Build history of the part. All positions in model axes, mm. Round coordinates to 2 decimals unless told otherwise and drop trailing zeros. Write each loop counter-clockwise with the first axis right and the second up, starting at its lowest first coordinate (ties: lowest second). Pieces come first, ordered by that corner, then holes. Notation, with made-up numbers: (3, 52.5) -> (33, 52.5) arc R28 cw to (33, 89.5) -> close; hole circle Ø10 at (77.5, 45). An arc over 180 degrees is marked (long way). Return JSON: item names as keys, results as strings.
from build123d import *

# Parameters (mm, degrees)
ESQUISSE1_W             = 10
ESQUISSE1_H             = 10
BOSS_EXTRU_1_DEPTH      = 30
ESQUISSE2_R             = 1.5
ENL_V_MAT_EXTRU_1_DEPTH = 30
CONG_1_R                = 0.5
ESQUISSE3_R             = 1.5
ENL_V_MAT_EXTRU_2_DEPTH = 10


with BuildPart() as part:
    # Esquisse1 → Boss.-Extru.1 (new body)
    with BuildSketch(Plane.XY):
        Rectangle(ESQUISSE1_W, ESQUISSE1_H)
    extrude(amount=BOSS_EXTRU_1_DEPTH)

    # Esquisse2 → Enlèv. mat.-Extru.1 (cut)
    with BuildSketch(Plane(origin=(5, 0, 0), x_dir=(0, 0, -1), z_dir=(1, 0, 0))):
        with Locations(Location((-3, -2, 0), (0, 0, 90))):
            Circle(ESQUISSE2_R)
    extrude(amount=-ENL_V_MAT_EXTRU_1_DEPTH, mode=Mode.SUBTRACT)

    # Congé1
    cong_1_edges = [part.edges().sort_by_distance(p)[0] for p in [
        (-5, 0, 30),
        (0, -5, 30),
        (5, 0, 30),
        (0, -5, 0),
        (-5, 0, 0),
        (0, 5, 0),
        (5, 0, 0),
        (5, -5, 15),
        (-5, -5, 15),
        (-5, 5, 15),
        (5, 5, 15),
        (0, 5, 30),
    ]]
    fillet(cong_1_edges, radius=CONG_1_R)

    # Esquisse3 → Enlèv. mat.-Extru.2 (cut)
    with BuildSketch(Plane.ZY.offset(5)):
        with Locations((27, -2)):
            Circle(ESQUISSE3_R)
    extrude(amount=-ENL_V_MAT_EXTRU_2_DEPTH, mode=Mode.SUBTRACT)


solid = part.part
Q1. Two-plate mould, pull along Y, no slides. Class faces 1 (the flat face through (5, 0, 15)), 2 (the cylindrical face through (0.07, -1.31, 1.67)), 3 (the cylindrical face through (-0.07, -1.93, 25.5)), 4 (the flat face through (0, 5, 15)): +Y half, -Y half, draft (parallel to the pull), parting line (faces both ways), or undercut.
Verdict:
{"face 1": "draft", "face 2": "undercut", "face 3": "undercut", "face 4": "+Y half"}
Q2. Saw through at B-B on z = 3. List the corners of the cut face in (x, y).
Verdict:
{"outline": "(-5, -4.5) arc R0.5 ccw to (-4.5, -5) -> (4.5, -5) arc R0.5 ccw to (5, -4.5) -> (5, -3.5) -> (-5, -3.5) -> close; (-5, -0.5) -> (5, -0.5) -> (5, 4.5) arc R0.5 ccw to (4.5, 5) -> (-4.5, 5) arc R0.5 ccw to (-5, 4.5) -> close"}
Q3. Saw through at A-A on y = -2. List the corners of the cut face in (x, z), then the cut area to 3 significant figures.
Verdict:
{"outline": "(-5, 0.5) arc R0.5 ccw to (-4.5, 0) -> (4.5, 0) arc R0.5 ccw to (5, 0.5) -> (5, 1.5) -> (-5, 1.5) -> close; (-5, 4.5) -> (5, 4.5) -> (5, 25.5) -> (-5, 25.5) -> close; (-5, 28.5) -> (5, 28.5) -> (5, 29.5) arc R0.5 ccw to (4.5, 30) -> (-4.5, 30) arc R0.5 ccw to (-5, 29.5) -> close", "area": "240 mm²"}
Q4. Saw through at C-C on x = 0.75. List the corners of the cut face in (y, z).
Verdict:
{"outline": "(-5, 0.5) arc R0.5 ccw to (-4.5, 0) -> (4.5, 0) arc R0.5 ccw to (5, 0.5) -> (5, 29.5) arc R0.5 ccw to (4.5, 30) -> (-4.5, 30) arc R0.5 ccw to (-5, 29.5) -> close; hole circle Ø3 at (-2, 3); hole circle Ø3 at (-2, 27)"}
Q5. Wall check: L1, parallel to Z at x = -0.5, y = -2.75; L2, parallel to Z at x = 1.75, y = -1.75; L3, parallel to Y at x = 2.5, z = 4. Give the ranges that are in metal, low to high.
Verdict:
{"L1": "z = 0 to 1.7, 4.3 to 25.7, 28.3 to 30", "L2": "z = 0 to 1.52, 4.48 to 25.52, 28.48 to 30", "L3": "y = -5 to -3.12, -0.88 to 5"}
